from build123d import *

# Parameters (mm, degrees)
F0_W      = 40
F0_H      = 40
F1_DEPTH  = 54.864
F2_R      = 10.16
F1_FACE_W = 19.68
F1_FACE_H = 19.68
F3_DEPTH  = 16.002


with BuildPart() as f1:
    # F0 (on Top) → F1 (new body)
    with BuildSketch(Plane.XY):
        with Locations((-12.078214, -3.62122)):
            Rectangle(F0_W, F0_H)
    extrude(amount=F1_DEPTH)

    # F2
    f2_edges = [f1.edges().sort_by_distance(p)[0] for p in [
        (-12.078214, -23.62122, 54.864),
        (7.921786, -3.62122, 54.864),
        (-12.078214, 16.37878, 54.864),
        (-32.078214, -3.62122, 54.864),
    ]]
    fillet(f2_edges, radius=F2_R)

    # F1_face (on face) → F3 (cut)
    with BuildSketch(Plane(origin=(-12.078214, -3.62122, 54.864), x_dir=(1, 0, 0), z_dir=(0, 0, 1))):
        Rectangle(F1_FACE_W, F1_FACE_H)
    extrude(amount=-F3_DEPTH, mode=Mode.SUBTRACT)


solid = f1.part
Source: CAD feature listing. Evaluate the final solid. Frame: model axes, mm. A direction names the side the tool comes from. Give positions to 0.01 mm unless a question says otherwise; leave off trailing zeros. Order: outer loops, then holes, each group sorted by start corner. A loop starts at its lowest first (then second) coordinate and runs counter-clockwise, first axis right, second up. Notation, with made-up numbers: (73.25, 20.25) -> (110.25, 20.25) arc R21 ccw to (110.25, 36.25) -> close; hole circle Ø3 at (44, 22.5). An arc over 180 degrees is marked (long way). Use a Markdown table: item, result.
1) Contact query for a flat-ended pin moving along its axis: P1, Ø10, axis at x = -8, y = -4.5, coming from the +Z side. Output: stop coordinate, or through.
Answer list:
| item | result |
|---|---|
| P1 | z = 38.86 |
2) Mould query, pull axis Y, two halves, no side actions, for faces 3 (the cylindrical face through (-11.798, -21.847, 50.44)), 4 (the flat face through (-12, -13.461, 47)), 5 (the cylindrical face through (-11.798, 14.605, 50.44)). Classes: +Y half, -Y half, draft (parallel to the pull), parting line (faces both ways), or undercut.
Answer list:
| item | result |
|---|---|
| face 3 | -Y half |
| face 4 | undercut |
| face 5 | +Y half |
3) Section query D-D, the plane z = 51. Return the cut outline in (x, y), then the cut area to 3 significant figures.
Answer list:
| item | result |
|---|---|
| outline | (-29.89, -21.44) -> (5.74, -21.44) -> (5.74, 14.19) -> (-29.89, 14.19) -> close; hole (-21.92, -13.46) -> (-2.24, -13.46) -> (-2.24, 6.22) -> (-21.92, 6.22) -> close |
| area | 882 mm² |
4) Section query B-B, the plane x = -5.5. Return the cut outline in (y, z), then the cut area to 3 significant figures.
Answer list:
| item | result |
|---|---|
| outline | (-23.62, 0) -> (16.38, 0) -> (16.38, 44.7) arc R10.16 ccw to (6.22, 54.86) -> (6.22, 38.86) -> (-13.46, 38.86) -> (-13.46, 54.86) arc R10.16 ccw to (-23.62, 44.7) -> close |
| area | 1,840 mm² |
5) Reachability of faces 1 (the flat face through (-12, 6.219, 47)), 2 (the flat face through (-12, -3, 0)) from +Z, -Z, +X, -X, +Y, -Y: full face, straight path, thin tool, end or side. Return the list, or none.
Answer list:
| item | result |
|---|---|
| face 1 | +Z |
| face 2 | -Z, +X, -X, +Y, -Y |
6) Section query A-A, the plane z = 41. Return the cut outline in (x, y).
Answer list:
| item | result |
|---|---|
| outline | (-32.08, -23.62) -> (7.92, -23.62) -> (7.92, 16.38) -> (-32.08, 16.38) -> close; hole (-21.92, -13.46) -> (-2.24, -13.46) -> (-2.24, 6.22) -> (-21.92, 6.22) -> close |
7) Section query C-C, the plane y = -9. Return the cut outline in (x, z).
Answer list:
| item | result |
|---|---|
| outline | (-32.08, 0) -> (7.92, 0) -> (7.92, 44.7) arc R10.16 ccw to (-2.24, 54.86) -> (-2.24, 38.86) -> (-21.92, 38.86) -> (-21.92, 54.86) arc R10.16 ccw to (-32.08, 44.7) -> close |
8) Ray query, line 1 along X through (y, z) = (-1, 39); line 2 along Z through (x, y) = (-9, -12); line 3 along Y through (x, z) = (-19, 49). Return the intervals inside material, ascending. Write a range as [from, to].
Answer list:
| item | result |
|---|---|
| line 1 | [-32.08, -21.92], [-2.24, 7.92] |
| line 2 | [0, 38.86] |
| line 3 | [-22.67, -13.46], [6.22, 15.43] |
